Source: CAD feature listing. Evaluate the final solid. Frame: model axes, mm. Give positions to 0.01 mm unless a question says otherwise; leave off trailing zeros. Write each loop counter-clockwise with the first axis right and the second up, starting at its lowest first coordinate (ties: lowest second). Pieces come first, ordered by that corner, then holes.
Autodesk Inventor part; units mm, degrees
ref_plane "YZ Plane" through (0, 0, 0) normal (1, 0, 0) x (0, 1, 0)
ref_plane "XZ Plane" through (0, 0, 0) normal (0, 1, 0) x (-1, 0, 0)
ref_plane "XY Plane" through (0, 0, 0) normal (0, 0, 1) x (1, 0, 0)
ref_plane "РабПлоскость1" through (0, 0, 0) normal (0, 0, 1) x (1, 0, 0)
sketch "Эскиз1" plane through (0, 0, 0) normal (0, 0, 1) x (1, 0, 0)
  line L0 (0.4175, 200.6086) -> (16.4175, 200.6086)
  line L1 (18.4175, 198.6086) -> (18.4175, 2.6086)
  line L2 (18.4175, 0.6086) -> (-1.5825, 0.6086)
  line L3 (-1.5825, 2.6086) -> (-1.5825, 198.6086)
  circle A0 centre (16.146, 17.8544) radius 1.1424
  circle A1 centre (16.1468, 2.552) radius 1.1415
  circle A2 centre (8.4175, 10.1937) radius 4.0638
  circle A3 centre (0.795, 2.6086) radius 1.0935
  circle A4 centre (0.7952, 17.8542) radius 1.0274
  line L4 (8.4175, 200.6086) -> (8.4175, 0.6086) construction
  arc A5 (18.4175, 0.6086) -> (18.4175, 2.6086) centre (16.6855, 1.6086) ccw
  arc A6 (-1.5825, 2.6086) -> (-1.5825, 0.6086) centre (0.1496, 1.6086) ccw
  circle A7 centre (8.3261, 183.6146) radius 1.1991
  circle A8 centre (15.4815, 190.7279) radius 1.1951
  circle A9 centre (8.3254, 197.9065) radius 1.1975
  circle A10 centre (1.0262, 190.7251) radius 1.1979
  circle A11 centre (8.3275, 190.7238) radius 4.2065
  arc A12 (0.4175, 200.6086) -> (-1.5825, 198.6086) centre (0.4175, 198.6086) ccw
  arc A13 (18.4175, 198.6086) -> (16.4175, 200.6086) centre (16.4175, 198.6086) ccw
  point P0 (18.4175, 0.6086)
  point P1 (18.4175, 200.6086)
  point P2 (-1.5825, 0.6086)
  dimension "d0" = 200
  dimension "d1" = 20
  dimension "d3" = 2
  dimension "d4" = 2
  dimension "d5" = 2
extrude "Выдавливание1" add sketch "Эскиз1" along normal blind 3
properties part number "рука"
1. Contact query for a flat-ended pin moving along its axis: P1, Ø1, axis at y = 139.5, z = 1.5, coming from the -X side. Output: stop coordinate, or through.
2. Line query: L1, parallel to Y at x = 16, z = 2.6; L2, parallel to Y at x = 5.5, z = 2.4; L3, parallel to Y at x = 7, z = 1.45. Output: solid intervals per line, ascending.
3. Cut plane A-A, the plane z = 0.65. State how many separate pieces and enclosed holes the cut face has, then the cut area to 3 significant figures.
4. Mould query, pull axis Y, two halves, no side actions, for faces 1 (the flat face through (8, 102, 0)), 2 (the cylindrical face through (4.358, 10.015, 1.479)). Classes: +Y half, -Y half, draft (parallel to the pull), parting line (faces both ways), or undercut.
5. Cut plane B-B, the plane y = 158. Return the cut outline in (x, z), then the cut area to 3 significant figures.
Response values:
1. P1: stops at x = -1.58
2. L1: y = 0.61 to 1.42, 3.68 to 16.72, 18.99 to 189.65, 191.8 to 200.61
2. L2: y = 0.61 to 7.36, 13.02 to 187.61, 193.84 to 200.61
2. L3: y = 0.61 to 6.39, 14 to 186.73, 194.72 to 200.61
3. separate pieces: 1
3. enclosed holes: 10
3. area: 3,860 mm2
4. face 1: draft
4. face 2: undercut
5. outline: (-1.58, 0) - (18.42, 0) - (18.42, 3) - (-1.58, 3) - close
5. area: 60.0 mm2
